from build123d import *

# Parameters (mm, degrees)
PAD009_DEPTH    = 49
THICKNESS002_T  = -3
SKETCH010_W     = 3
SKETCH010_H     = 3
POCKET_DEPTH    = 98.001
SKETCH011_R     = 2
POCKET001_DEPTH = 3
SKETCH012_R     = 2
POCKET002_DEPTH = 3
SKETCH013_R     = 2
POCKET003_DEPTH = 3


with BuildPart() as part:
    # Sketch009 → Pad009 (new body, symmetric)
    with BuildSketch(Plane.YZ):
        Polygon((0, 0), (-209, 0), (-209, 10), (-142, 30), (-67, 30), (0, 10), align=None)
    extrude(amount=PAD009_DEPTH, both=True)

    # Thickness002
    thickness002_openings = [part.faces().sort_by_distance(p)[0] for p in [
        (49, -104.5, 12.734956),
        (0, -104.5, 0),
        (-49, -104.5, 12.734956),
    ]]
    offset(amount=THICKNESS002_T, openings=thickness002_openings)

    # Sketch010 (on Face6 of Thickness002) → Pocket (cut, through all)
    with BuildSketch(Plane.YZ.offset(49)):
        with Locations((-1.5, 1.5)):
            Rectangle(SKETCH010_W, SKETCH010_H)
    extrude(amount=-POCKET_DEPTH, mode=Mode.SUBTRACT)

    # Sketch011 (on Face3 of Pocket) → Pocket001 (cut)
    with BuildSketch(Plane(origin=(0, -19.8404581714, 66.4655348742), x_dir=(1, 0, 0), z_dir=(0, -0.2860355264, 0.9582190134))):
        with Locations((-20, -142.4467263242)):
            Circle(SKETCH011_R)
        with Locations((20, -142.4467263242)):
            Circle(SKETCH011_R)
        with Locations((20, -182.4467263242)):
            Circle(SKETCH011_R)
        with Locations((-20, -182.4467263242)):
            Circle(SKETCH011_R)
    extrude(amount=-POCKET001_DEPTH, mode=Mode.SUBTRACT)

    # Sketch012 (on Face7 of Pocket001) → Pocket002 (cut)
    with BuildSketch(Plane.XY.offset(30)):
        with Locations((-20, -124.5)):
            Circle(SKETCH012_R)
        with Locations((20, -124.5)):
            Circle(SKETCH012_R)
        with Locations((-20, -84.5)):
            Circle(SKETCH012_R)
        with Locations((20, -84.5)):
            Circle(SKETCH012_R)
    extrude(amount=-POCKET002_DEPTH, mode=Mode.SUBTRACT)

    # Sketch013 (on Face13 of Pocket002) → Pocket003 (cut)
    with BuildSketch(Plane(origin=(0, 2.7408467989, 9.1818367764), x_dir=(1, 0, 0), z_dir=(0, 0.2860355264, 0.9582190134))):
        with Locations((-20, -17.8210474767)):
            Circle(SKETCH013_R)
        with Locations((20, -17.8210474767)):
            Circle(SKETCH013_R)
        with Locations((20, -57.8210474767)):
            Circle(SKETCH013_R)
        with Locations((-20, -57.8210474767)):
            Circle(SKETCH013_R)
    extrude(amount=-POCKET003_DEPTH, mode=Mode.SUBTRACT)


solid = part.part
Can you work these out from the model? Positions are in its coordinate system, mm. A direction names the side the tool comes from. Coordinates: 2 decimals unless noted, no trailing zeros. Loops run counter-clockwise (first coordinate to the right, second up) from the corner with the lowest first, then second, coordinate; pieces in that order, holes last. Notation, with made-up numbers: (38.25, 16.25) - (75.25, 16.25) arc R33 cw to (75.25, 44.25) - close; hole circle Ø8 at (84.25, 8). An arc over 180 degrees is marked (long way). Put each result on its own line as item: value. Start each with the question number.
Item 1: If we mould it in two halves opening along X, with no side actions, what happens to faces 3 (the face through (-49, -104, 27.3)), 4 (the face through (-21.474, -154.617, 24.69)), 5 (the face through (0.69, -174.23, 17.25))? For each: +X half, -X half, draft (parallel to the pull), parting line (faces both ways), or undercut.
Item 2: Suppose I cut it at D-D (y = -151.5). Please give me the cut outline in (x, z), and give its area (3 significant figures).
Item 3: Which directions (+Z, -Z, +X, -X, +Y, -Y) give clear straight access to the entire face, cutting with the end or side of a thin tool? Please do faces 1 (the face through (1, -3, 5)), 2 (the face through (18.41, -54.25, 24.65)).
Item 4: If I drill on line 1 along Y through (x, z) = (-15.5, 6.25); line 2 along Z through (x, y) = (-30.5, -95); line 3 along Z through (x, y) = (19, -184), over which ranges is the centre line in solid material (lowest first)?
Item 5: For pin 1 (2 mm diameter, centred on y = -181.5, z = 19.5, fed in from -X); pin 2 (4.5 mm diameter, centred on x = 20, y = -84.5, fed in from +Z); pin 3 (10 mm diameter, centred on x = -38, y = -128.5, fed in from -Z); pin 4 (2.5 mm diameter, centred on x = 13, y = -2, fed in from -Z), each with a flat end and sliding along its axis, tell me the tip position at first contact or that it passes through.
Item 6: Suppose I cut it at B-B (x = -32). Please give me the cut outline in (y, z), and give its area (3 significant figures).
Item 7: Suppose I cut it at A-A (y = -84.5). Please give me the cut outline in (x, z), and give its area (3 significant figures).
Item 8: Suppose I cut it at C-C (x = -20). State how many separate pieces and enclosed holes the cut face has, and give its area (3 significant figures).
Here are the results:
1. face 3: -X half
1. face 4: undercut
1. face 5: draft
2. outline: (-49, 24.03) - (49, 24.03) - (49, 27.16) - (-49, 27.16) - close
2. area: 307 mm²
3. face 1: -Z, +X, -X
3. face 2: none
4. line 1: -209 to -206, -3 to 0
4. line 2: 27 to 30
4. line 3: 14.33 to 17.46
5. pin 1: through
5. pin 2: z = 30
5. pin 3: z = 27
5. pin 4: z = 3
6. outline: (-209, 0) - (-206, 0) - (-206, 7.76) - (-141.56, 27) - (-67.44, 27) - (-3, 7.76) - (-3, 3) - (0, 3) - (0, 10) - (-67, 30) - (-142, 30) - (-209, 10) - close
6. area: 679 mm²
7. outline: (-49, 27) - (-22, 27) - (-22, 30) - (-49, 30) - close; (-18, 27) - (18, 27) - (18, 30) - (-18, 30) - close; (22, 27) - (49, 27) - (49, 30) - (22, 30) - close
7. area: 270 mm²
8. separate pieces: 7
8. enclosed holes: 0
8. area: 607 mm²
